from build123d import *

# Parameters (mm, degrees)
BOSS_EXTRUDE1_DEPTH        = 58
SKETCH2_OUTSIDE_W          = 147.986
SKETCH2_OUTSIDE_H          = 126.948
TAB_AND_SLOT_CONTOUR_DEPTH = 3
MOUNTING_TAB_SLOT_REACH    = 197.382
SKETCH4_W                  = 10.2
SKETCH4_H                  = 4.48444402
EYE_APERTURE_REACH         = 197.382
SKETCH3_RX                 = 26.778256145
SKETCH3_RY                 = 15


with BuildPart() as part:
    # Sketch1 → Boss-Extrude1 (new, symmetric)
    with BuildSketch(Plane.XY):
        Polygon((-66.659178779, 221.764297559), (-69.478256642, 222.790357989), (-101.297584098, 135.367474301), (-98.478506236, 134.341413871), align=None)
    extrude(amount=BOSS_EXTRUDE1_DEPTH, both=True)

    # Sketch2 outside → tab and slot contour (cut)
    with BuildSketch(Plane(origin=(-132.954285367, 48.391402392, 0), x_dir=(0, 0, 1), z_dir=(-0.9396926207859096, 0.34202014332566527, 0))):
        with Locations((0, 139.075)):
            Rectangle(SKETCH2_OUTSIDE_W, SKETCH2_OUTSIDE_H)
        with BuildLine():
            Line((57.97107056, 98.09508485), (49, 181.128574477))
            ThreePointArc((49, 181.128574477), (47.369183029, 184.312070804), (44.02892944, 185.59149209))
            Line((44.02892944, 185.59149209), (-44.02892944, 185.59149209))
            ThreePointArc((-44.02892944, 185.59149209), (-47.369183029, 184.312070804), (-49, 181.128574477))
            Line((-49, 181.128574477), (-57.97107056, 98.09508485))
            ThreePointArc((-57.97107056, 98.09508485), (-56.720578714, 94.217748875), (-53, 92.558002463))
            Line((-53, 92.558002463), (53, 92.558002463))
            ThreePointArc((53, 92.558002463), (56.720578714, 94.217748875), (57.97107056, 98.09508485))
        make_face(mode=Mode.SUBTRACT)
    extrude(amount=-TAB_AND_SLOT_CONTOUR_DEPTH, mode=Mode.SUBTRACT)

    # Sketch4 → mounting tab slot (cut, up to next)
    with BuildSketch(Plane(origin=(-132.954285367, 48.391402392, 0), x_dir=(0, 0, 1), z_dir=(-0.9396926207859096, 0.3420201433256655, 0)), mode=Mode.PRIVATE) as mounting_tab_slot_sk1:
        with Locations((-25, 172.357359377)):
            Rectangle(SKETCH4_W, SKETCH4_H)
    mounting_tab_slot_tool1 = extrude(mounting_tab_slot_sk1.sketch, amount=-MOUNTING_TAB_SLOT_REACH, mode=Mode.PRIVATE) & part.part
    # Sketch4 → mounting tab slot (cut, up to next)
    with BuildSketch(Plane(origin=(-132.954285367, 48.391402392, 0), x_dir=(0, 0, 1), z_dir=(-0.9396926207859096, 0.3420201433256655, 0)), mode=Mode.PRIVATE) as mounting_tab_slot_sk2:
        with Locations((-25, 102.516403068)):
            Rectangle(SKETCH4_W, SKETCH4_H)
    mounting_tab_slot_tool2 = extrude(mounting_tab_slot_sk2.sketch, amount=-MOUNTING_TAB_SLOT_REACH, mode=Mode.PRIVATE) & part.part
    # Sketch4 → mounting tab slot (cut, up to next)
    with BuildSketch(Plane(origin=(-132.954285367, 48.391402392, 0), x_dir=(0, 0, 1), z_dir=(-0.9396926207859096, 0.3420201433256655, 0)), mode=Mode.PRIVATE) as mounting_tab_slot_sk3:
        with Locations((25, 172.357359377)):
            Rectangle(SKETCH4_W, SKETCH4_H)
    mounting_tab_slot_tool3 = extrude(mounting_tab_slot_sk3.sketch, amount=-MOUNTING_TAB_SLOT_REACH, mode=Mode.PRIVATE) & part.part
    # Sketch4 → mounting tab slot (cut, up to next)
    with BuildSketch(Plane(origin=(-132.954285367, 48.391402392, 0), x_dir=(0, 0, 1), z_dir=(-0.9396926207859096, 0.3420201433256655, 0)), mode=Mode.PRIVATE) as mounting_tab_slot_sk4:
        with Locations((25, 102.516403068)):
            Rectangle(SKETCH4_W, SKETCH4_H)
    mounting_tab_slot_tool4 = extrude(mounting_tab_slot_sk4.sketch, amount=-MOUNTING_TAB_SLOT_REACH, mode=Mode.PRIVATE) & part.part
    add(mounting_tab_slot_tool1.solids().sort_by_distance((-74.004597, 210.354341, -25))[0], mode=Mode.SUBTRACT)
    add(mounting_tab_slot_tool2.solids().sort_by_distance((-97.89161, 144.72531, -25))[0], mode=Mode.SUBTRACT)
    add(mounting_tab_slot_tool3.solids().sort_by_distance((-74.004597, 210.354341, 25))[0], mode=Mode.SUBTRACT)
    add(mounting_tab_slot_tool4.solids().sort_by_distance((-97.89161, 144.72531, 25))[0], mode=Mode.SUBTRACT)

    # Sketch3 → eye aperture (cut, up to next)
    with BuildSketch(Plane(origin=(-132.954285367, 48.391402392, 0), x_dir=(0, 0, 1), z_dir=(-0.9396926207859096, 0.3420201433256652, 0)), mode=Mode.PRIVATE) as eye_aperture_sk1:
        with Locations(Location((-27, 138.436881223), (0, 0, -90))):
            Ellipse(SKETCH3_RX, SKETCH3_RY)
    eye_aperture_tool1 = extrude(eye_aperture_sk1.sketch, amount=-EYE_APERTURE_REACH, mode=Mode.PRIVATE) & part.part
    # Sketch3 → eye aperture (cut, up to next)
    with BuildSketch(Plane(origin=(-132.954285367, 48.391402392, 0), x_dir=(0, 0, 1), z_dir=(-0.9396926207859096, 0.3420201433256652, 0)), mode=Mode.PRIVATE) as eye_aperture_sk2:
        with Locations(Location((27, 138.436881223), (0, 0, -90))):
            Ellipse(SKETCH3_RX, SKETCH3_RY)
    eye_aperture_tool2 = extrude(eye_aperture_sk2.sketch, amount=-EYE_APERTURE_REACH, mode=Mode.PRIVATE) & part.part
    add(eye_aperture_tool1.solids().sort_by_distance((-85.606083, 178.479518, -27))[0], mode=Mode.SUBTRACT)
    add(eye_aperture_tool2.solids().sort_by_distance((-85.606083, 178.479518, 27))[0], mode=Mode.SUBTRACT)


solid = part.part
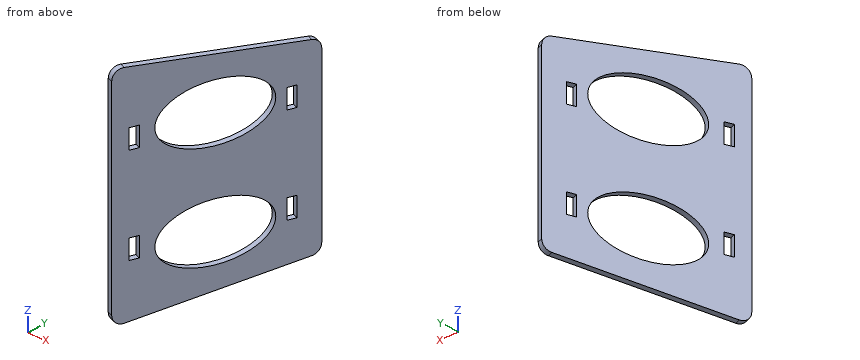
Can you work these out from the model? Positions are in its coordinate system, mm. Give positions to 0.01 mm unless a question says otherwise; leave off trailing zeros. Write each loop counter-clockwise with the first axis right and the second up, starting at its lowest first coordinate (ties: lowest second). Pieces come first, ordered by that corner, then holes. Notation, with made-up numbers: (48, -25) -> (92, -25) arc R33 cw to (92, 6) -> close; hole circle Ø8 at (37.25, 71). An arc over 180 degrees is marked (long way). Answer as a JSON object with one key per item and string values. Group by question number.
Item 1: I'm going to push flat-ended pins straight in: P1, Ø3.5, axis at x = -97, y = 145, coming from the -Z side; P2, Ø3.5, axis at x = -72.5, y = 209, coming from the -Z side; P3, Ø2, axis at x = -95.5, y = 144.5, coming from the -Z side; P4, Ø1.5, axis at x = -76, y = 189, coming from the +Z side. Where does each tip first touch, or does it pass through?
Item 2: Suppose I cut it at B-B (y = 179). State how many separate pieces and enclosed holes the cut face has, plus the area to 3 significant figures.
Item 3: Please list where these lines run through material, in increasing order: line 1 (Z direction, x = -71.5, y = 215); line 2 (X direction, y = 204.5, z = -38); line 3 (X direction, y = 150, z = 22.5). Write a range as [from, to].
Item 4: Suppose I cut it at A-A (z = 3). Please give me the cut outline in (x, y), plus the area to 3 significant figures.
Findings:
{
 "1": {"P1": "stops at z = -57.62", "P2": "stops at z = -50.22", "P3": "stops at z = -57.54", "P4": "passes through"},
 "2": {"separate pieces": "3", "enclosed holes": "0", "area": "150 mm²"},
 "3": {"line 1": "z = [-49.38, 49.38]", "line 2": "x = [-76.14, -72.94]", "line 3": "x = [-95.97, -92.78]"},
 "4": {"outline": "(-101.3, 135.37) -> (-98.48, 134.34) -> (-66.66, 221.76) -> (-69.48, 222.79) -> close", "area": "279 mm²"}
}
